The listing builds one solid part. Answer for the finished solid, in the listing's coordinates (mm). Face numbers are marked on the shaded views. A direction names the side the tool comes from. Give positions to 0.01 mm unless a question says otherwise; leave off trailing zeros. Loops run counter-clockwise (first coordinate to the right, second up) from the corner with the lowest first, then second, coordinate; pieces in that order, holes last. Notation, with made-up numbers: (46.5, 64) - (70.5, 64) arc R30 ccw to (70.5, 101) - close; hole circle Ø9 at (32, -1.75). An arc over 180 degrees is marked (long way). Answer as CSV lines item,"result". Start each with the question number.
1) Find the intervals of material crossed by line 1 along Z through (x, y) = (78.7, 34); line 2 along X through (y, z) = (35, -48); line 3 along Y through (x, z) = (41, -74.5), in increasing order.
2) A cutting plane is placed at C-C (z = 0). Determine the outline of the cut face in (x, y), and give its area (3 significant figures).
3) A cutting plane is placed at B-B (x = -62.5). Determine the outline of the cut face in (y, z).
4) A cutting plane is placed at A-A (z = 87.5). Determine the outline of the cut face in (x, y), and give its area (4 significant figures).
5) A flat-ended cylindrical pin translates along its axis: pin 1 (4 mm diameter, centred on x = -57, z = -19, fed in from +Y). Find the tip coordinate at first contact, or state that the pin passes through.
6) For the marked faces 1 and 2, determine the directions among +Z, -Z, +X, -X, +Y, -Y from which every point of the face is accessible in a straight line to the end or side of a thin tool.
7) A cutting plane is placed at D-D (z = -105). Determine the outline of the cut face in (x, y).
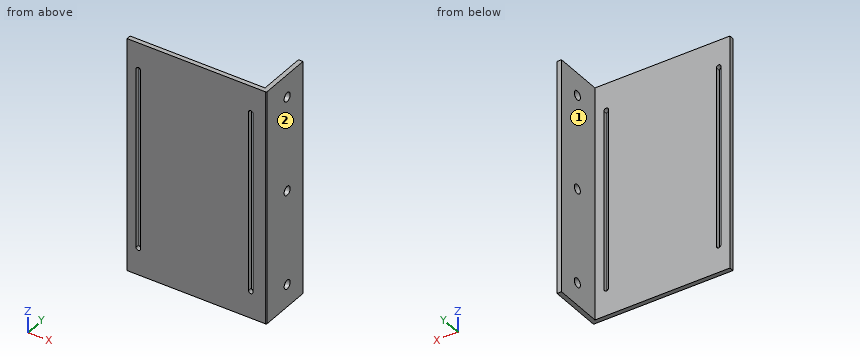
```python
from build123d import *

# Parameters (mm, degrees)
F0_W      = 150
F0_H      = 260
F1_DEPTH  = 5
F3_DEPTH  = 6
F5_DEPTH  = 6
F6_DEPTH  = 6
F7_DEPTH  = 6
F8_DEPTH  = 6
F9_W      = 60
F9_H      = 260
F10_DEPTH = 5
F11_R     = 5
F12_DEPTH = 6
F13_R     = 1


with BuildPart() as f1:
    # F0 (on Front) → F1 (new body)
    with BuildSketch(Plane.XZ):
        Rectangle(F0_W, F0_H)
    extrude(amount=-F1_DEPTH)

    # F2 (on face) → F3 (cut)
    with BuildSketch(Plane.XZ):
        with BuildLine():
            ThreePointArc((-60, 100), (-62.5, 102.5), (-65, 100))
            Line((-65, 100), (-60, 100))
        make_face()
        with BuildLine():
            ThreePointArc((-60, 100), (-62.5, 97.5), (-65, 100))
            Line((-65, 100), (-65, -100))
            ThreePointArc((-65, -100), (-62.5, -97.5), (-60, -100))
            Line((-60, -100), (-60, 100))
        make_face()
        with BuildLine():
            Line((-60, 100), (-65, 100))
            ThreePointArc((-65, 100), (-62.5, 97.5), (-60, 100))
        make_face()
        with BuildLine():
            ThreePointArc((-60, -100), (-62.5, -97.5), (-65, -100))
            Line((-65, -100), (-60, -100))
        make_face()
        with BuildLine():
            Line((-60, -100), (-65, -100))
            ThreePointArc((-65, -100), (-62.5, -102.5), (-60, -100))
        make_face()
    extrude(amount=-F3_DEPTH, mode=Mode.SUBTRACT)

    # F4 (on face) → F5 (cut)
    with BuildSketch(Plane.XZ):
        with BuildLine():
            ThreePointArc((65, 100), (62.5, 102.5), (60, 100))
            Line((60, 100), (65, 100))
        make_face()
        with BuildLine():
            ThreePointArc((65, 100), (62.5, 97.5), (60, 100))
            Line((60, 100), (60, -100))
            ThreePointArc((60, -100), (62.5, -97.5), (65, -100))
            Line((65, -100), (65, 100))
        make_face()
        with BuildLine():
            Line((65, 100), (60, 100))
            ThreePointArc((60, 100), (62.5, 97.5), (65, 100))
        make_face()
        with BuildLine():
            ThreePointArc((65, -100), (62.5, -97.5), (60, -100))
            Line((60, -100), (65, -100))
        make_face()
        with BuildLine():
            Line((65, -100), (60, -100))
            ThreePointArc((60, -100), (62.5, -102.5), (65, -100))
        make_face()
    extrude(amount=-F5_DEPTH, mode=Mode.SUBTRACT)

    # F4 (on face) → F6 (cut)
    with BuildSketch(Plane.XZ):
        with BuildLine():
            ThreePointArc((65, 100), (62.5, 102.5), (60, 100))
            Line((60, 100), (65, 100))
        make_face()
        with BuildLine():
            ThreePointArc((65, 100), (62.5, 97.5), (60, 100))
            Line((60, 100), (60, -100))
            ThreePointArc((60, -100), (62.5, -97.5), (65, -100))
            Line((65, -100), (65, 100))
        make_face()
        with BuildLine():
            Line((65, 100), (60, 100))
            ThreePointArc((60, 100), (62.5, 97.5), (65, 100))
        make_face()
        with BuildLine():
            ThreePointArc((65, -100), (62.5, -97.5), (60, -100))
            Line((60, -100), (65, -100))
        make_face()
        with BuildLine():
            Line((65, -100), (60, -100))
            ThreePointArc((60, -100), (62.5, -102.5), (65, -100))
        make_face()
    extrude(amount=-F6_DEPTH, mode=Mode.SUBTRACT)

    # F2 (on face) → F7 (cut)
    with BuildSketch(Plane.XZ):
        with BuildLine():
            ThreePointArc((-60, 100), (-62.5, 102.5), (-65, 100))
            Line((-65, 100), (-60, 100))
        make_face()
        with BuildLine():
            ThreePointArc((-60, 100), (-62.5, 97.5), (-65, 100))
            Line((-65, 100), (-65, -100))
            ThreePointArc((-65, -100), (-62.5, -97.5), (-60, -100))
            Line((-60, -100), (-60, 100))
        make_face()
        with BuildLine():
            Line((-60, 100), (-65, 100))
            ThreePointArc((-65, 100), (-62.5, 97.5), (-60, 100))
        make_face()
        with BuildLine():
            ThreePointArc((-60, -100), (-62.5, -97.5), (-65, -100))
            Line((-65, -100), (-60, -100))
        make_face()
        with BuildLine():
            Line((-60, -100), (-65, -100))
            ThreePointArc((-65, -100), (-62.5, -102.5), (-60, -100))
        make_face()
    extrude(amount=-F7_DEPTH, mode=Mode.SUBTRACT)

    # F4 (on face) → F8 (cut)
    with BuildSketch(Plane.XZ):
        with BuildLine():
            ThreePointArc((65, 100), (62.5, 102.5), (60, 100))
            Line((60, 100), (65, 100))
        make_face()
        with BuildLine():
            ThreePointArc((65, 100), (62.5, 97.5), (60, 100))
            Line((60, 100), (60, -100))
            ThreePointArc((60, -100), (62.5, -97.5), (65, -100))
            Line((65, -100), (65, 100))
        make_face()
        with BuildLine():
            Line((65, 100), (60, 100))
            ThreePointArc((60, 100), (62.5, 97.5), (65, 100))
        make_face()
        with BuildLine():
            ThreePointArc((65, -100), (62.5, -97.5), (60, -100))
            Line((60, -100), (65, -100))
        make_face()
        with BuildLine():
            Line((65, -100), (60, -100))
            ThreePointArc((60, -100), (62.5, -102.5), (65, -100))
        make_face()
    extrude(amount=-F8_DEPTH, mode=Mode.SUBTRACT)

    # F9 (on face) → F10 (join)
    with BuildSketch(Plane.YZ.offset(75)):
        with Locations((30, 0)):
            Rectangle(F9_W, F9_H)
    extrude(amount=F10_DEPTH)

    # F11 (on face) → F12 (cut)
    with BuildSketch(Plane.YZ.offset(80)):
        with Locations((34, 0)):
            Circle(F11_R)
        with Locations((34, 105)):
            Circle(F11_R)
        with Locations((34, -105)):
            Circle(F11_R)
    extrude(amount=-F12_DEPTH, mode=Mode.SUBTRACT)

    # F13
    f13_edges = [f1.edges().sort_by_distance(p)[0] for p in [
        (80, 0, 0),
    ]]
    fillet(f13_edges, radius=F13_R)


solid = f1.part
```
Ans:
1,line 1,"-130 to -110, -100 to -5, 5 to 100, 110 to 130"
1,line 2,"75 to 80"
1,line 3,"0 to 5"
2,outline,"(-75, 0) - (-65, 0) - (-65, 5) - (-75, 5) - close; (-60, 0) - (60, 0) - (60, 5) - (-60, 5) - close; (65, 0) - (79, 0) arc R1 ccw to (80, 1) - (80, 29) - (75, 29) - (75, 5) - (65, 5) - close; (75, 39) - (80, 39) - (80, 60) - (75, 60) - close"
2,area,"950 mm2"
3,outline,"(0, -130) - (5, -130) - (5, -102.5) - (0, -102.5) - close; (0, 102.5) - (5, 102.5) - (5, 130) - (0, 130) - close"
4,outline,"(-75, 0) - (-65, 0) - (-65, 5) - (-75, 5) - close; (-60, 0) - (60, 0) - (60, 5) - (-60, 5) - close; (65, 0) - (79, 0) arc R1 ccw to (80, 1) - (80, 60) - (75, 60) - (75, 5) - (65, 5) - close"
4,area,"1,000 mm2"
5,pin 1,"y = 5"
6,face 1,"+Z, -Z, -X, +Y"
6,face 2,"+Z, -Z, +X, +Y, -Y"
7,outline,"(-75, 0) - (79, 0) arc R1 ccw to (80, 1) - (80, 29) - (75, 29) - (75, 5) - (-75, 5) - close; (75, 39) - (80, 39) - (80, 60) - (75, 60) - close"
